For this review, take the finished solid that the model builds, in its own axes (mm). A direction names the side the tool comes from. Round coordinates to 2 decimals unless told otherwise and drop trailing zeros. Loops run counter-clockwise (first coordinate to the right, second up) from the corner with the lowest first, then second, coordinate; pieces in that order, holes last. Notation, with made-up numbers: (-21, 12.25) -> (33, 12.25) arc R10 cw to (33, 20.25) -> close; hole circle Ø9 at (15, 50). An arc over 180 degrees is marked (long way). One line per question, with ' | ' between items. Start each with the question number.
1. Consider section A-A (x = 18). Write out the cut boundary in (y, z).
2. Consider section C-C (y = 18.5). Write out the cut boundary in (x, z) (3 decimals), and give its area (3 significant figures).
3. Wall thickness on line 1 along Z through (x, y) = (12, 133); line 2 along Y through (x, z) = (-19.5, 40); line 3 along Y through (x, z) = (18.5, 28.5): over which ranges is each line inside the solid? List them lowest first.
4. For faces 1 (the face through (0, 102, 6.35)), 2 (the face through (0, 6, 76.2)), list the 3-axis set-ups (+Z, -Z, +X, -X, +Y, -Y) from which the entire face can be reached by the end or side of a thin tool; tool diameter is ignored.
5. For pin 1 Ø4 at (x, y) = (7, 27) entering from +Z; pin 2 Ø13.5 at (x, y) = (-11, 122.5) entering from +Z; pin 3 Ø1.5 at (x, z) = (6, 25.5) entering from +Y, all flat-tipped, find the tip position at first contact; note any pin that passes through.
6. Consider section B-B (z = 27). Write out the cut boundary in (x, y) (3 decimals), and give its area (3 significant figures).
```python
from build123d import *

# Parameters (mm, degrees)
BOSS_EXTRUDE1_DEPTH = 22.225
CHAMFER1_SIZE       = 25.4


with BuildPart() as part:
    # Sketch1 → Boss-Extrude1 (new, symmetric)
    with BuildSketch(Plane(origin=(0, 0, 0), x_dir=(0, 0, -1), z_dir=(1, 0, 0))):
        Polygon((0, 0), (0, 165.1), (-6.35, 165.1), (-6.35, 12.7), (-76.2, 12.7), (-76.2, 0), align=None)
    extrude(amount=BOSS_EXTRUDE1_DEPTH, both=True)

    # Chamfer1
    chamfer1_edges = [part.edges().sort_by_distance(p)[0] for p in [
        (0, 12.7, 6.35),
    ]]
    chamfer(chamfer1_edges, length=CHAMFER1_SIZE)


solid = part.part
```
Answer block:
1) outline: (0, 0) -> (165.1, 0) -> (165.1, 6.35) -> (38.1, 6.35) -> (12.7, 31.75) -> (12.7, 76.2) -> (0, 76.2) -> close
2) outline: (-22.225, 0) -> (22.225, 0) -> (22.225, 25.95) -> (-22.225, 25.95) -> close | area: 1,150 mm2
3) line 1: z = 0 to 6.35 | line 2: y = 0 to 12.7 | line 3: y = 0 to 15.95
4) face 1: +Z, +X, -X, +Y | face 2: +Z, +X, -X, +Y, -Y
5) pin 1: stops at z = 19.45 | pin 2: stops at z = 6.35 | pin 3: stops at y = 19.7
6) outline: (-22.225, 0) -> (22.225, 0) -> (22.225, 17.45) -> (-22.225, 17.45) -> close | area: 776 mm2
